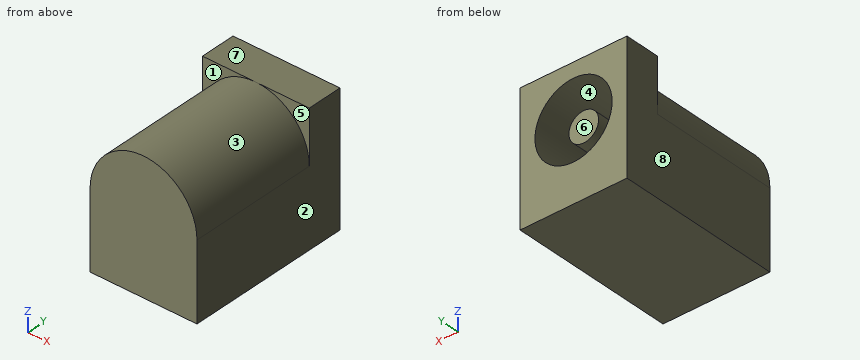
from build123d import *

# Parameters (mm, degrees)
SKETCH1_W           = 9
SKETCH1_H           = 3
BOSS_EXTRUDE1_DEPTH = 11
BOSS_EXTRUDE2_DEPTH = 11
SKETCH3_R           = 3.25
CUT_EXTRUDE1_DEPTH  = 13
SKETCH4_R           = 1.25
BOSS_EXTRUDE3_DEPTH = 12


with BuildPart() as part:
    # Sketch1 → Boss-Extrude1 (new body)
    with BuildSketch(Plane.XY):
        with Locations((0, 1.5)):
            Rectangle(SKETCH1_W, SKETCH1_H)
    extrude(amount=BOSS_EXTRUDE1_DEPTH)

    # Sketch2 → Boss-Extrude2 (add)
    with BuildSketch(Plane.XZ):
        with BuildLine():
            Line((-4.5, 0), (4.5, 0))
            Line((4.5, 0), (4.5, 6.5))
            ThreePointArc((4.5, 6.5), (0, 11), (-4.5, 6.5))
            Line((-4.5, 6.5), (-4.5, 0))
        make_face()
    extrude(amount=BOSS_EXTRUDE2_DEPTH)

    # Sketch3 → Cut-Extrude1 (cut)
    with BuildSketch(Plane(origin=(0, 3, 0), x_dir=(1, 0, 0), z_dir=(0, 1, 0))):
        with Locations(Location((0, -6.5, 0), (0, 0, 180))):
            Circle(SKETCH3_R)
    extrude(amount=-CUT_EXTRUDE1_DEPTH, mode=Mode.SUBTRACT)

    # Sketch4 → Boss-Extrude3 (add)
    with BuildSketch(Plane(origin=(0, -10, 0), x_dir=(1, 0, 0), z_dir=(0, 1, 0))):
        with Locations((0, -6.5)):
            Circle(SKETCH4_R)
    extrude(amount=BOSS_EXTRUDE3_DEPTH)


solid = part.part
Geometry check sheet. Reference: the model listing, model coordinates, mm. Face numbers are marked on the shaded views. A direction names the side the tool comes from. Give positions to 0.01 mm unless a question says otherwise; leave off trailing zeros. Write each loop counter-clockwise with the first axis right and the second up, starting at its lowest first coordinate (ties: lowest second). Pieces come first, ordered by that corner, then holes. Notation, with made-up numbers: M 29.5,-29.5 L 67.5,-29.5 A20 ccw 67.5,1.5 Z; hole C 54.5,34 d6. An arc over 180 degrees is marked long. One line per question, with ' | ' between items.
1. Cross-section at D-D (x = 3). Enter the section's corners in (y, z).
Ans:
outline: M -11,0 L 3,0 L 3,5.25 L -10,5.25 L -10,7.75 L 3,7.75 L 3,11 L 0,11 L 0,9.85 L -11,9.85 Z
2. Scan lines: line 1 along Z through (x, y) = (0, -4.25); line 2 along X through (y, z) = (-7.75, 7); line 3 along X through (y, z) = (-3.5, 5.5). Record each from-to range of solid material in increasing order. Write a range as from..to.
Ans:
line 1: 0..3.25, 5.25..7.75, 9.75..11 | line 2: -4.47..-3.21, -1.15..1.15, 3.21..4.47 | line 3: -4.5..-3.09, -0.75..0.75, 3.09..4.5
3. Gauge pin test, flat end, axial feed: pin 1 (1.2 mm diameter, centred on x = 0, z = 6, fed in from +Y). Record the tip position at first contact, or that the pin passes through.
Ans:
pin 1: y = 2
4. Cross-section at A-A (y = -2.25). Enter the section's corners in (x, z).
Ans:
outline: M -4.5,0 L 4.5,0 L 4.5,6.5 A4.5 ccw -4.5,6.5 Z; C 0,6.5 d2.5; hole C 0,6.5 d6.5
5. Mould release check, pull along Z, two halves, no side actions. Record for the marked faces 6, 7 and 8: released by +Z, released by -Z, zero draft, split by the parting line, or undercut.
Ans:
face 6: undercut | face 7: released by +Z | face 8: zero draft
6. Cross-section at B-B (z = 9.5). Enter the section's corners in (x, y).
Ans:
outline: M -4.5,0 L -3.35,0 L -3.35,-11 L 3.35,-11 L 3.35,0 L 4.5,0 L 4.5,3 L 1.25,3 L 1.25,-10 L -1.25,-10 L -1.25,3 L -4.5,3 Z
7. Set-up check for the marked faces 1, 2, 3, 4 and 5: record each of +Z, -Z, +X, -X, +Y, -Y from which the full face is reachable in a straight line by a thin tool's end or side.
Ans:
face 1: +Z, -X, -Y | face 2: +Z, -Z, +X, +Y, -Y | face 3: +Z, -Y | face 4: +Y | face 5: +Z, +X, -Y
